Check sheet for the modelled part. Datum: model origin and axes. Units: mm. Round coordinates to 2 decimals unless told otherwise and drop trailing zeros. Write each loop counter-clockwise with the first axis right and the second up, starting at its lowest first coordinate (ties: lowest second). Pieces come first, ordered by that corner, then holes. Notation, with made-up numbers: (42, 29.5) - (53, 29.5) arc R22 ccw to (53, 59.5) - close; hole circle Ø5 at (28, -3.5). An arc over 180 degrees is marked (long way). Answer as a JSON object with one key per item and string values. Group by question number.
Item 1: Sectioned sample at B-B on z = 5.75. Record the boundary of the cut face in (x, y), plus the area to 3 significant figures.
Item 2: Sectioned sample at A-A on y = 0.3. Record the boundary of the cut face in (x, z).
Item 3: Sectioned sample at C-C on x = 3.5. Record the boundary of the cut face in (y, z), plus the area to 3 significant figures.
Item 4: Thickness scan on line 1 (Z direction, x = -1.5, y = 0.3); line 2 (X direction, y = 0.35, z = 6.75); line 3 (Z direction, x = -2.5, y = 0.3). Record the ranges inside material, lowest first.
Autodesk Inventor part; units mm, degrees
ref_plane "shtrmnl_XY" through (0, 0, 0) normal (0, 1, 0) x (1, 0, 0)
ref_plane "shtrmnl_YZ" through (0, 0, 0) normal (1, 0, 0) x (0, 0, -1)
ref_plane "shtrmnl_ZX" through (0, 0, 0) normal (0, 0, -1) x (0, 1, 0)
sketch "Sketch_1" plane through (0, 0, 0) normal (0, 1, 0) x (-1, 0, 0)
  line L0 (4.7244, 3.9497) -> (3.2385, 3.9497)
  line L1 (3.2385, 3.9497) -> (3.2385, 6.1468)
  arc A0 (3.2385, 6.1468) -> (1.8415, 6.1468) centre (2.54, 6.1468) ccw
  line L2 (1.8415, 6.1468) -> (1.8415, 3.9497)
  line L3 (1.8415, 3.9497) -> (-1.8415, 3.9497)
  line L4 (-1.8415, 3.9497) -> (-1.8415, 6.1468)
  arc A1 (-1.8415, 6.1468) -> (-3.2385, 6.1468) centre (-2.54, 6.1468) ccw
  line L5 (-3.2385, 6.1468) -> (-3.2385, 3.9497)
  line L6 (-3.2385, 3.9497) -> (-4.7244, 3.9497)
  line L7 (-4.7244, 3.9497) -> (-4.7244, -3.9497)
  line L8 (-4.7244, -3.9497) -> (4.7244, -3.9497)
  line L9 (4.7244, -3.9497) -> (4.7244, 3.9497)
extrude "Extrusion1" add sketch "Sketch_1" along normal blind 0.4064
ref_plane "shtrmnl_XY" through (0, 0, 0) normal (0, 1, 0) x (1, 0, 0)
ref_plane "shtrmnl_YZ" through (0, 0, 0) normal (1, 0, 0) x (0, 0, -1)
ref_plane "shtrmnl_ZX" through (0, 0, 0) normal (0, 0, -1) x (0, 1, 0)
properties part number "M201230TX-switch"
Completed:
{
 "1": {"outline": "(-3.24, 0) - (-1.84, 0) - (-1.84, 0.41) - (-3.24, 0.41) - close; (1.84, 0) - (3.24, 0) - (3.24, 0.41) - (1.84, 0.41) - close", "area": "1.14 mm²"},
 "2": {"outline": "(-4.72, -3.95) - (4.72, -3.95) - (4.72, 3.95) - (3.24, 3.95) - (3.24, 6.15) arc R0.7 ccw to (1.84, 6.15) - (1.84, 3.95) - (-1.84, 3.95) - (-1.84, 6.15) arc R0.7 ccw to (-3.24, 6.15) - (-3.24, 3.95) - (-4.72, 3.95) - close"},
 "3": {"outline": "(0, -3.95) - (0.41, -3.95) - (0.41, 3.95) - (0, 3.95) - close", "area": "3.21 mm²"},
 "4": {"line 1": "-3.95 to 3.95", "line 2": "-2.89 to -2.19, 2.19 to 2.89", "line 3": "-3.95 to 6.84"}
}
